Source: three-view drawing plus pictorial views. Frame: mm from the lowest corner of the part. Give positions to 0.01 mm unless a question says otherwise; leave off trailing zeros. Order: outer loops, then holes, each group sorted by start corner. A loop starts at its lowest first (then second) coordinate and runs counter-clockwise, first axis right, second up. Notation, with made-up numbers: (66.25, 48.5) -> (118.25, 48.5) arc R25 ccw to (118.25, 82.5) -> close; hole circle Ø3 at (47.5, 26.5). An arc over 180 degrees is marked (long way). Answer in a Markdown table with one row per item. Add a question column.
Q1. Line query: line 1 along Y through (x, z) = (23, 3.05); line 2 along Y through (x, z) = (23, 2.65); line 3 along Z through (x, y) = (40, 43). Output: solid intervals per line, ascending. Write a range as from..to.
Q2. Cut plane D-D on y = 29. Return the cut outline in (x, z), and give its area (3 significant figures).
Q3. Cut plane A-A on y = 23. Return the cut outline in (x, z), and give its area (3 significant figures).
Q4. Cut plane C-C on z = 2.4. Return the cut outline in (x, y).
Q5. Contact query for flat-ended pins moving along their axis: P1, Ø3, axis at x = 23, y = 23, coming from the -Z side; P2, Ø2, axis at x = 33, y = 33.5, coming from the +Z side. Output: stop coordinate, or through.
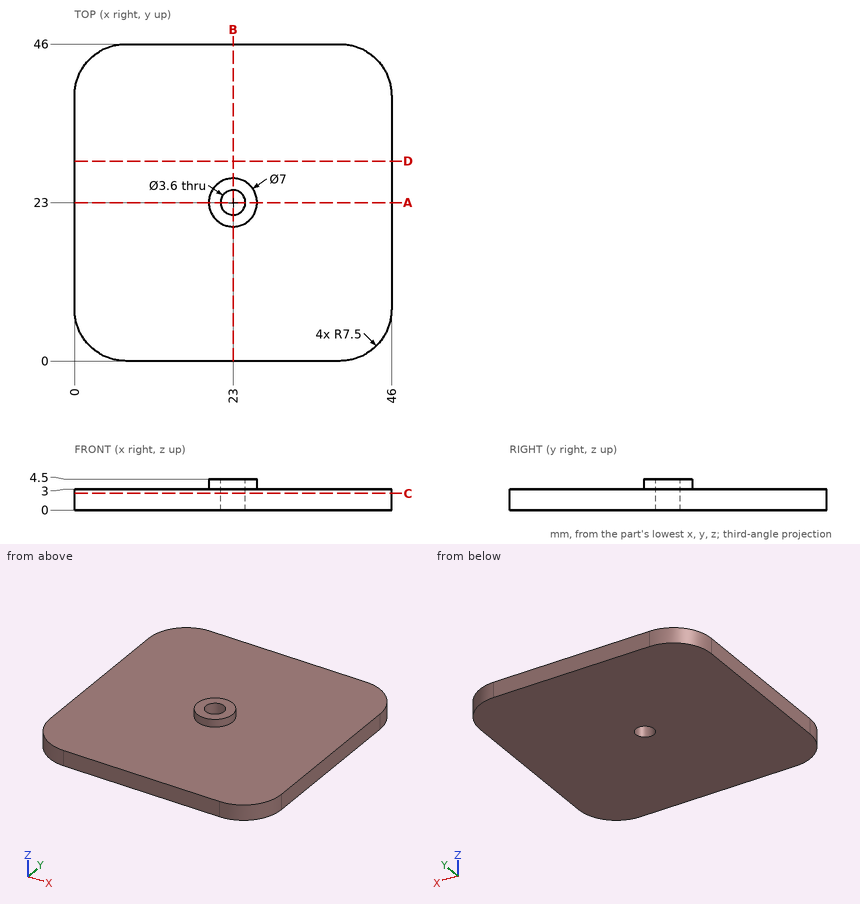
Completed:
| question | item | result |
|---|---|---|
| 1 | line 1 | y = 19.5..21.2, 24.8..26.5 |
| 1 | line 2 | y = 0..21.2, 24.8..46 |
| 1 | line 3 | z = 0..3 |
| 2 | outline | (0, 0) -> (46, 0) -> (46, 3) -> (0, 3) -> close |
| 2 | area | 138 mm² |
| 3 | outline | (0, 0) -> (21.2, 0) -> (21.2, 4.5) -> (19.5, 4.5) -> (19.5, 3) -> (0, 3) -> close; (24.8, 0) -> (46, 0) -> (46, 3) -> (26.5, 3) -> (26.5, 4.5) -> (24.8, 4.5) -> close |
| 3 | area | 132 mm² |
| 4 | outline | (0, 7.5) arc R7.5 ccw to (7.5, 0) -> (38.5, 0) arc R7.5 ccw to (46, 7.5) -> (46, 38.5) arc R7.5 ccw to (38.5, 46) -> (7.5, 46) arc R7.5 ccw to (0, 38.5) -> close; hole circle Ø3.6 at (23, 23) |
| 5 | P1 | passes through |
| 5 | P2 | stops at z = 3 |
